```python
from build123d import *

# Parameters (mm, degrees)
F0_R     = 18.35
F0_R_2   = 7.1
F1_DEPTH = 24
F3_DEPTH = 24
F4_SIZE  = 1
F5_SIZE2 = 1
F5_SIZE  = 1
F6_R     = 1


with BuildPart() as f1:
    # F0 (on Top) → F1 (new body)
    with BuildSketch(Plane.XY):
        Circle(F0_R)
        Circle(F0_R_2, mode=Mode.SUBTRACT)
    extrude(amount=F1_DEPTH)

    # F2 (on face) → F3 (join)
    with BuildSketch(Plane.XY.offset(24)):
        with BuildLine():
            ThreePointArc((4.9907414279, 5.05), (0, 7.1), (-4.9907414279, 5.05))
            Line((-4.9907414279, 5.05), (4.9907414279, 5.05))
        make_face()
    extrude(amount=-F3_DEPTH)

    # F4
    f4_edges = [f1.edges().sort_by_distance(p)[0] for p in [
        (0, 5.05, 24),
        (0, -7.1, 24),
    ]]
    chamfer(f4_edges, length=F4_SIZE)

    # F5
    f5_edges = [f1.edges().sort_by_distance(p)[0] for p in [
        (0, 5.05, 0),
        (0, -7.1, 0),
    ]]
    chamfer(f5_edges, length=F5_SIZE, length2=F5_SIZE2)

    # F6
    f6_edges = [f1.edges().sort_by_distance(p)[0] for p in [
        (-18.35, 0, 24),
    ]]
    fillet(f6_edges, radius=F6_R)


solid = f1.part
```
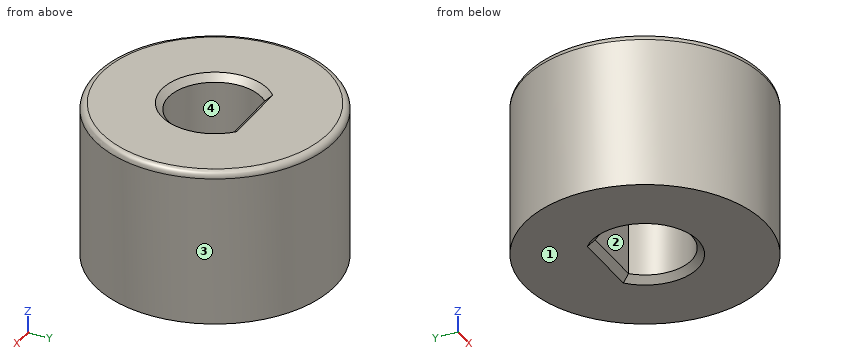
Design review of the part built by this model. Coordinates are the model's own, in mm. Face numbers are marked on the shaded views. Coordinates: 2 decimals unless noted, no trailing zeros. Order: outer loops, then holes, each group sorted by start corner. A loop starts at its lowest first (then second) coordinate and runs counter-clockwise, first axis right, second up. Notation, with made-up numbers: (79.5, 64) -> (137.5, 64) arc R28 ccw to (137.5, 103) -> close; hole circle Ø6 at (-7.5, 0). An arc over 180 degrees is marked (long way). One line per item, written item: value. Start each with the question number.
Q1. For probe 1 along Y at (x, z) = (0, 5.5); probe 2 along Y at (x, z) = (6.5, 20); probe 3 along X at (y, z) = (-6, 20), list the stretches that pass through material, from the lowest coordinate up.
Q2. Mouldability with a two-part tool opening along Y and no side actions: class the marked faces 1, 2, 3 and 4 as pulls with the +Y half, pulls with the -Y half, needs draft (parallel to the pull), parting line crosses it, or undercut.
Q3. Insertion check: pin 1 Ø4 at (y, z) = (-11.5, 17) entering from +X; pin 2 Ø1 at (x, z) = (5.5, 20.5) entering from -Y; pin 3 Ø10 at (y, z) = (-10, 19) entering from -X. Each pin has a flat end and moves straight along its axis. Give the tip position at first contact, or say it passes through.
Q4. Take a section at B-B, the plane z = 15. State the section outline as (x, y) points.
Q5. Take a section at A-A, the plane x = 0. State the section outline as (y, z) points, then the cut area to 3 significant figures.
Values follow:
1. probe 1: y = -18.35 to -7.1, 5.05 to 18.35
1. probe 2: y = -17.16 to -2.86, 2.86 to 17.16
1. probe 3: x = -17.34 to -3.8, 3.8 to 17.34
2. face 1: needs draft
2. face 2: undercut
2. face 3: parting line crosses it
2. face 4: undercut
3. pin 1: stops at x = 15.7
3. pin 2: stops at y = -17.66
3. pin 3: stops at x = -17.66
4. outline: circle Ø36.7 at (0, 0); hole (-4.99, 5.05) arc R7.1 ccw (long way) to (4.99, 5.05) -> close
5. outline: (-18.35, 0) -> (-8.1, 0) -> (-7.1, 1) -> (-7.1, 23) -> (-8.1, 24) -> (-17.35, 24) arc R1 ccw to (-18.35, 23) -> close; (5.05, 1) -> (6.05, 0) -> (18.35, 0) -> (18.35, 23) arc R1 ccw to (17.35, 24) -> (6.05, 24) -> (5.05, 23) -> close
5. area: 587 mm2
